For this review, take the finished solid that the model builds, in its own axes (mm). A direction names the side the tool comes from. Coordinates: 2 decimals unless noted, no trailing zeros. Loops run counter-clockwise (first coordinate to the right, second up) from the corner with the lowest first, then second, coordinate; pieces in that order, holes last. Notation, with made-up numbers: M 52.25,86.5 L 70.25,86.5 A16 cw 70.25,110.5 Z; hole C -37,4 d10. An arc over 180 degrees is marked long. Put each result on its own line as item: value.
```python
from build123d import *

# Parameters (mm, degrees)
BOSS_EXTRUDE1_DEPTH = 5
SKETCH3_W           = 2
SKETCH3_H           = 5.099019514
CUT_EXTRUDE3_DEPTH  = 2


with BuildPart() as part:
    # Sketch1 → Boss-Extrude1 (new body)
    with BuildSketch(Plane.XY):
        Polygon((0, 0), (-2, 0), (-4, -1), (-4, 1), (-2, 3), (-2, 4), (0, 4), (0, 3), (2, 1), (2, -1), align=None)
    extrude(amount=BOSS_EXTRUDE1_DEPTH)

    # Sketch3 → Cut-Extrude3 (cut)
    with BuildSketch(Plane(origin=(0, 0, 0), x_dir=(-1, 0, 0), z_dir=(0, -0.980580676, 0.196116135))):
        with Locations((1, -2.549509757)):
            Rectangle(SKETCH3_W, SKETCH3_H)
    extrude(amount=CUT_EXTRUDE3_DEPTH, mode=Mode.SUBTRACT)


solid = part.part
```
(1) Tool access review of faces 5 (the flat face through (1, -0.5, 2.5)), 6 (the flat face through (-1, 0.5, 2.5)), 7 (the flat face through (0, 3.5, 2.5)): name each direction out of +Z, -Z, +X, -X, +Y, -Y from which nothing blocks a thin tool from reaching the whole face with its end or side.
Determined:
face 5: +Z, -Z, -Y
face 6: +Z, -Y
face 7: +Z, -Z, +X, +Y
(2) Add section D-D (x = 0.4). Write out the cut boundary in (y, z).
Determined:
outline: M -0.2,0 L 2.6,0 L 2.6,5 L -0.2,5 Z
(3) Add section B-B (z = 4.45). Write out the cut boundary in (x, y), plus the area to 3 significant figures.
Determined:
outline: M -4,-1 L -2,0 L -2,0.89 L 0,0.89 L 0,0 L 2,-1 L 2,1 L 0,3 L 0,4 L -2,4 L -2,3 L -4,1 Z
area: 16.2 mm^2
(4) Draft analysis for pull direction X (two halves, no side actions). For faces 1 (the flat face through (-1, 2, 5)), 2 (the flat face through (0, 0.3, 3.2)), 3 (the flat face through (1, 2, 2)), 4 (the flat face through (-3, -0.5, 2.5)), state which applies: +X half, -X half, draft (parallel to the pull), parting line (faces both ways), or undercut.
Determined:
face 1: draft
face 2: undercut
face 3: +X half
face 4: undercut
(5) Wall thickness on line 1 along X through (y, z) = (3.75, 0.35); line 2 along X through (y, z) = (-0.2, 4.8); line 3 along X through (y, z) = (1.8, 4.6): over which ranges is each line inside the solid? List them lowest first. Write a range as [from, to].
Determined:
line 1: x = [-2, 0]
line 2: x = [-4, -2.4], [0.4, 2]
line 3: x = [-3.2, 1.2]
(6) Add section A-A (y = -0.4). Write out the cut boundary in (x, z).
Determined:
outline: M -4,0 L -2.8,0 L -2.8,5 L -4,5 Z; M 0.8,0 L 2,0 L 2,5 L 0.8,5 Z
(7) For pin 1 (1.1 mm diameter, centred on y = 3.5, z = 3, fed in from +X); pin 2 (0.5 mm diameter, centred on y = 3.5, z = 3, fed in from -X), all flat-tipped, find the tip position at first contact; note any pin that passes through.
Determined:
pin 1: stops at x = 0.05
pin 2: stops at x = -2
(8) Add section C-C (y = 0.2). Write out the cut boundary in (x, z).
Determined:
outline: M -4,0 L 2,0 L 2,5 L 0,5 L 0,1 L -2,1 L -2,5 L -4,5 Z
